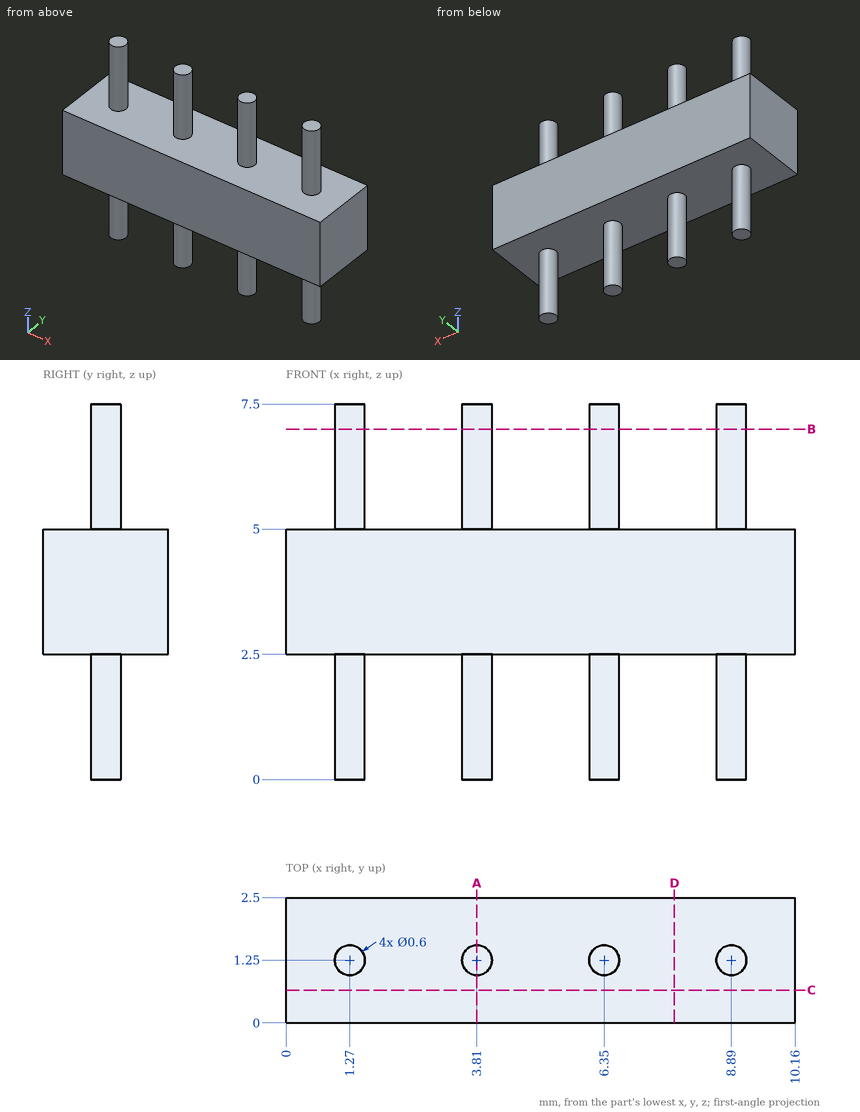
Answer from the drawing. Dimensions are ordinates in mm from the lowest x, y and z of the part. Give positions to 0.01 mm unless a question says otherwise; leave off trailing zeros. Loops run counter-clockwise (first coordinate to the right, second up) from the corner with the lowest first, then second, coordinate; pieces in that order, holes last. Notation, with made-up numbers: (28.5, -1.75) - (85.5, -1.75) arc R19 ccw to (85.5, 21.25) - close; hole circle Ø9 at (-20, -39.75). An arc over 180 degrees is marked (long way). Answer as a JSON object with one key per item and string values.
1. A cutting plane is placed at D-D (x = 7.75). Write down the section's boundary in (y, z), then the cut area to 3 significant figures.
Determined:
{"outline": "(0, 2.5) - (2.5, 2.5) - (2.5, 5) - (0, 5) - close", "area": "6.25 mm²"}
2. Find the intervals of material crossed by L1, parallel to Z at x = 7.75, y = 0.7; L2, parallel to X at y = 1.4, z = 1; L3, parallel to X at y = 1.05, z = 6, in increasing order. Write a range as [from, to].
Determined:
{"L1": "[2.5, 5]", "L2": "[1.01, 1.53], [3.55, 4.07], [6.09, 6.61], [8.63, 9.15]", "L3": "[1.05, 1.49], [3.59, 4.03], [6.13, 6.57], [8.67, 9.11]"}
3. A cutting plane is placed at B-B (z = 7). Write down the section's boundary in (x, y).
Determined:
{"outline": "circle Ø0.6 at (1.27, 1.25); circle Ø0.6 at (3.81, 1.25); circle Ø0.6 at (6.35, 1.25); circle Ø0.6 at (8.89, 1.25)"}
4. A cutting plane is placed at C-C (y = 0.65). Write down the section's boundary in (x, z), then the cut area to 3 significant figures.
Determined:
{"outline": "(0, 2.5) - (10.16, 2.5) - (10.16, 5) - (0, 5) - close", "area": "25.4 mm²"}
5. A cutting plane is placed at A-A (x = 3.81). Write down the section's boundary in (y, z).
Determined:
{"outline": "(0, 2.5) - (0.95, 2.5) - (0.95, 0) - (1.55, 0) - (1.55, 2.5) - (2.5, 2.5) - (2.5, 5) - (1.55, 5) - (1.55, 7.5) - (0.95, 7.5) - (0.95, 5) - (0, 5) - close"}
